Build history of the part. All positions in model axes, mm. A direction names the side the tool comes from. Round coordinates to 2 decimals unless told otherwise and drop trailing zeros. Order: outer loops, then holes, each group sorted by start corner. A loop starts at its lowest first (then second) coordinate and runs counter-clockwise, first axis right, second up. Notation, with made-up numbers: M 43.5,-10.75 L 54.5,-10.75 A33 cw 54.5,26.25 Z; hole C 78.5,27 d6. An arc over 180 degrees is marked long. Use CSV: the item, a comma, the result in double quotes.
from build123d import *

# Parameters (mm, degrees)
F2_R     = 3.175
F3_DEPTH = 5.54365


with BuildPart() as f1:
    # F0 (on Front) → F1 (revolve)
    with BuildSketch(Plane.XZ):
        Polygon((0, 8.62508), (0, 18.142857), (-39.37, 18.142857), (-39.37, 12.599207), (-26.67, 12.599207), (-26.67, 4.938889), (-26.67, 0), (-13.97, 0), (-13.97, 8.62508), (-7.62, 8.62508), (-7.62, 4.81508), (-5.08, 4.81508), (-5.08, 8.62508), align=None)
    revolve(axis=Axis((0, 0, 21.598651), (0, 0, -1)))

    # F2 (on face) → F3 (cut, through all)
    with BuildSketch(Plane.XY.offset(18.142857)):
        with Locations((0, 31.75)):
            Circle(F2_R)
        with Locations((31.75, 0)):
            Circle(F2_R)
        with Locations((0, -31.75)):
            Circle(F2_R)
        with Locations((-31.75, 0)):
            Circle(F2_R)
    extrude(amount=-F3_DEPTH, mode=Mode.SUBTRACT)


solid = f1.part
(1) Cut at A-A, the plane y = 0. Give the cut face in (x, z) (3 decimals).
Answer block:
outline,"M -39.37,12.599 L -34.925,12.599 L -34.925,18.143 L -39.37,18.143 Z; M -28.575,12.599 L -26.67,12.599 L -26.67,0 L -13.97,0 L -13.97,8.625 L -7.62,8.625 L -7.62,4.815 L -5.08,4.815 L -5.08,8.625 L 5.08,8.625 L 5.08,4.815 L 7.62,4.815 L 7.62,8.625 L 13.97,8.625 L 13.97,0 L 26.67,0 L 26.67,12.599 L 28.575,12.599 L 28.575,18.143 L -28.575,18.143 Z; M 34.925,12.599 L 39.37,12.599 L 39.37,18.143 L 34.925,18.143 Z"
(2) Cut at D-D, the plane x = -33. Give the cut face in (y, z), and give its area (3 significant figures).
Answer block:
outline,"M -21.47,12.6 L -2.92,12.6 L -2.92,18.14 L -21.47,18.14 Z; M 2.92,12.6 L 21.47,12.6 L 21.47,18.14 L 2.92,18.14 Z"
area,"206 mm²"
(3) Drop flat-ended pins along their axis: pin 1 (5 mm diameter, centred on x = 19, z = 3, fed in from +Y); pin 2 (11.5 mm diameter, centred on x = 0, y = 0, fed in from -Z); pin 3 (2 mm diameter, centred on x = -0.5, z = 13, fed in from -Y); pin 4 (5.5 mm diameter, centred on x = 0, y = -31.75, fed in from -Z). Give the stop position or say it passes through.
Answer block:
pin 1,"stops at y = 20.95"
pin 2,"stops at z = 4.82"
pin 3,"stops at y = -39.37"
pin 4,"passes through"
(4) Cut at C-C, the plane z = 13.75. Give the cut face in (x, y) (3 decimals).
Answer block:
outline,"C 0,0 d78.74; hole C -31.75,0 d6.35; hole C 0,-31.75 d6.35; hole C 0,31.75 d6.35; hole C 31.75,0 d6.35"
(5) Wall check: line 1 (X direction, y = 1, z = 13); line 2 (Z direction, x = 7.5, y = 34); line 3 (X direction, y = -3, z = 1.75). Give the ranges that are in metal, low to high. Write a range as from..to.
Answer block:
line 1,"x = -39.36..-34.76, -28.74..28.74, 34.76..39.36"
line 2,"z = 12.6..18.14"
line 3,"x = -26.5..-13.64, 13.64..26.5"
(6) Cut at B-B, the plane y = 31.75. Give the cut face in (x, z) (3 decimals).
Answer block:
outline,"M -23.279,12.599 L -3.175,12.599 L -3.175,18.143 L -23.279,18.143 Z; M 3.175,12.599 L 23.279,12.599 L 23.279,18.143 L 3.175,18.143 Z"
(7) Tool access for faces 4 (the face through (-0.69, -34.85, 15.41)), 5 (the face through (0, 0, 8.625)): list every direction of +Z, -Z, +X, -X, +Y, -Y with a clear straight run to the whole face (end or side of a thin tool).
Answer block:
face 4,"+Z, -Z"
face 5,"-Z"
(8) Two-plate mould, pull along X, no slides. Class faces 1 (the face through (-0.69, 28.65, 15.41)), 2 (the face through (-11, -11, 0)), 3 (the face through (3.472, 26.443, 6.211)): released by +X, released by -X, zero draft, split by the parting line, or undercut.
Answer block:
face 1,"undercut"
face 2,"zero draft"
face 3,"split by the parting line"
